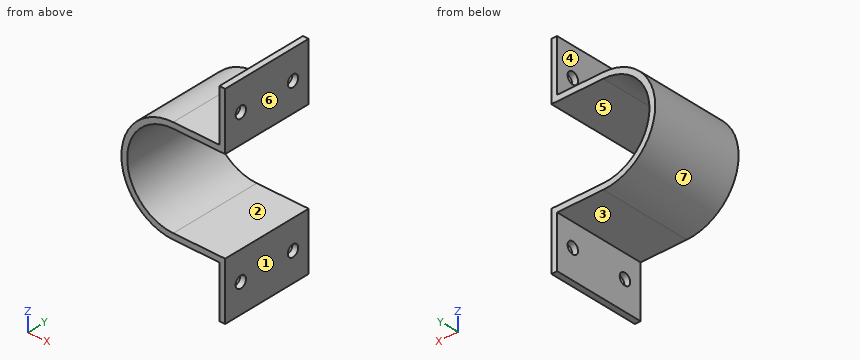
Autodesk Inventor part; units mm, degrees
ref_plane "YZ Plane" through (0, 0, 0) normal (1, 0, 0) x (0, 1, 0)
ref_plane "XZ Plane" through (0, 0, 0) normal (0, 1, 0) x (-1, 0, 0)
ref_plane "XY Plane" through (0, 0, 0) normal (0, 0, 1) x (1, 0, 0)
sketch "Sketch1" plane through (0, 0, 0) normal (0, 1, 0) x (-1, 0, 0)
  arc A0 (0, -20) -> (0, 20) centre (0, 0) ccw
  arc A1 (0, -22.5) -> (0, 22.5) centre (0, 0) ccw
  line L0 (0, 22.5) -> (-20, 22.5)
  line L1 (-22.5, 20) -> (-20, 20)
  line L2 (-20, 22.5) -> (-20, 45)
  line L3 (-20, 45) -> (-22.5, 45)
  line L4 (-22.5, 45) -> (-22.5, 20)
  line L5 (8.3208, 0) -> (-8.3208, 0)
  line L6 (0, 20) -> (-22.5, 20)
  line L7 (0, -22.5) -> (-20, -22.5)
  line L8 (-22.5, -20) -> (-20, -20)
  line L9 (-20, -22.5) -> (-20, -45)
  line L10 (-20, -45) -> (-22.5, -45)
  line L11 (-22.5, -45) -> (-22.5, -20)
  line L12 (0, -20) -> (-22.5, -20)
  point P0 (-22.5, 22.5)
  point P1 (-22.5, -22.5)
  dimension "d0" = 40
  dimension "d1" = 2.5
  dimension "d2" = 25
extrude "Extrusion1" add sketch "Sketch1" along normal blind 40
sketch "Sketch2" plane through (22.5, 0, 45) normal (1, 0, 0) x (0, 0, -1)
  line L0 (12.5, 32.5) -> (77.5, 32.5)
  line L1 (77.5, 32.5) -> (77.5, 7.5)
  line L2 (77.5, 7.5) -> (12.5, 7.5)
  line L3 (12.5, 7.5) -> (12.5, 32.5)
  line L4 (0, 0) -> (0, 40)
  line L5 (25, 40) -> (65, 40)
  circle A0 centre (12.5, 32.5) radius 2.5
  circle A1 centre (77.5, 32.5) radius 2.5
  circle A2 centre (77.5, 7.5) radius 2.5
  circle A3 centre (12.5, 7.5) radius 2.5
  point P0 (45, 0)
  dimension "d5" = 65
  dimension "d6" = 25
  dimension "d7" = 12.5
  dimension "d8" = 7.5
  dimension "d9" = 5
  dimension "d10" = 5
  dimension "d11" = 5
  dimension "d12" = 5
extrude "Extrusion2" cut sketch "Sketch2" against normal blind 40 contours L3 A0 L0 | L0 A0 L3 | A1 L1 L0 | L0 L1 A1 | A3 L2 L3 | L3 L2 A3 | A2 L2 L1 | L1 L2 A2
properties part number "steeringbracket"
Check sheet for the modelled part. Datum: model origin and axes. Units: mm. Face numbers are marked on the shaded views. A direction names the side the tool comes from. Round coordinates to 2 decimals unless told otherwise and drop trailing zeros. Order: outer loops, then holes, each group sorted by start corner. A loop starts at its lowest first (then second) coordinate and runs counter-clockwise, first axis right, second up. Notation, with made-up numbers: (85, 7.25) - (96, 7.25) arc R22 cw to (96, 27.25) - close; hole circle Ø3 at (66, -28). An arc over 180 degrees is marked (long way). Write item = value, one per line.
Q1. Section check C-C (z = 32.5). Record the boundary of the cut face in (x, y).
Computed:
outline = (20, 0) - (22.5, 0) - (22.5, 5) - (20, 5) - close; (20, 10) - (22.5, 10) - (22.5, 30) - (20, 30) - close; (20, 35) - (22.5, 35) - (22.5, 40) - (20, 40) - close
Q2. Go/stop test with flat-tipped pins: pin 1 (1 mm diameter, centred on y = 28.5, z = -7.5, fed in from -X); pin 2 (12 mm diameter, centred on x = -11.5, z = -1.5, fed in from -Y); pin 3 (12 mm diameter, centred on y = 27.5, z = 11, fed in from +X); pin 4 (2 mm diameter, centred on x = -3, y = 21, fed in from +Z). Record where each tip stops, or that it passes through.
Computed:
pin_1 = -21.38
pin_2 = through
pin_3 = -10.54
pin_4 = 22.41
Q3. Section check B-B (y = 32.5). Record the boundary of the cut face in (x, z).
Computed:
outline = (0, -22.5) - (20, -22.5) - (20, -30) - (22.5, -30) - (22.5, -20) - (0, -20) arc R20 cw to (0, 20) - (22.5, 20) - (22.5, 30) - (20, 30) - (20, 22.5) - (0, 22.5) arc R22.5 ccw to start; (20, -45) - (22.5, -45) - (22.5, -35) - (20, -35) - close; (20, 35) - (22.5, 35) - (22.5, 45) - (20, 45) - close
Q4. Thickness scan on line 1 along Y through (x, z) = (21.55, -32.5); line 2 along Z through (x, y) = (21.55, 32.5); line 3 along Y through (x, z) = (21, -32). Record the ranges inside material, lowest first.
Computed:
line_1 = 0 to 5, 10 to 30, 35 to 40
line_2 = -45 to -35, -30 to -20, 20 to 30, 35 to 45
line_3 = 0 to 5.05, 9.95 to 30.05, 34.95 to 40
Q5. Tool access check on the marked faces 1, 2, 3 and 4. Record the directions out of +Z, -Z, +X, -X, +Y, -Y that give a thin tool (end or side, any length) a straight path to the whole face; none if there is none.
Computed:
face_1 = +Z, -Z, +X, +Y, -Y
face_2 = +X, +Y, -Y
face_3 = -Z, -X, +Y, -Y
face_4 = +Z, -X, +Y, -Y
Q6. Section check A-A (x = 10.5). Record the boundary of the cut face in (y, z).
Computed:
outline = (0, -22.5) - (40, -22.5) - (40, -20) - (0, -20) - close; (0, 20) - (40, 20) - (40, 22.5) - (0, 22.5) - close
Q7. Section check D-D (y = 11). Record the boundary of the cut face in (x, z).
Computed:
outline = (0, -22.5) - (20, -22.5) - (20, -45) - (22.5, -45) - (22.5, -20) - (0, -20) arc R20 cw to (0, 20) - (22.5, 20) - (22.5, 45) - (20, 45) - (20, 22.5) - (0, 22.5) arc R22.5 ccw to start
Q8. Draft check along Z on the marked faces 5, 6 and 7. Enter one of: pulls with the +Z half, pulls with the -Z half, needs draft (parallel to the pull), parting line crosses it, or undercut.
Computed:
face_5 = undercut
face_6 = needs draft
face_7 = parting line crosses it
